The model under review builds one solid part; all positions refer to its coordinate system, in mm. Face numbers are marked on the shaded views. A direction names the side the tool comes from. Coordinates: 2 decimals unless noted, no trailing zeros. Loops run counter-clockwise (first coordinate to the right, second up) from the corner with the lowest first, then second, coordinate; pieces in that order, holes last. Notation, with made-up numbers: M 30,55.5 L 87,55.5 A23 cw 87,81.5 Z; hole C 7.5,-29.75 d9. An arc over 180 degrees is marked long. Return JSON: item names as keys, results as strings.
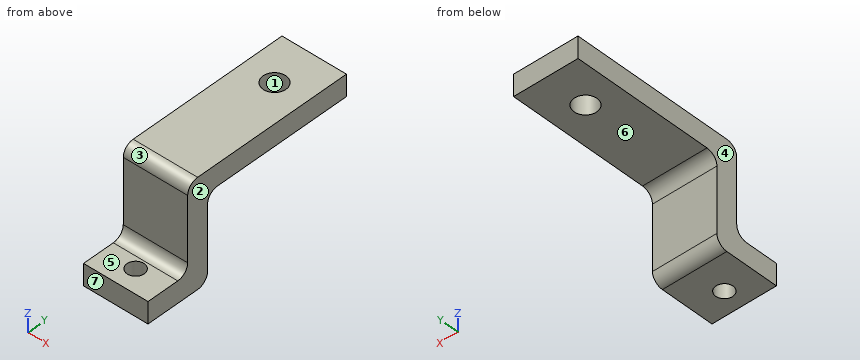
Autodesk Inventor part; units mm, degrees
ref_plane "YZ Plane" through (0, 0, 0) normal (1, 0, 0) x (0, 1, 0)
ref_plane "XZ Plane" through (0, 0, 0) normal (0, 1, 0) x (-1, 0, 0)
ref_plane "XY Plane" through (0, 0, 0) normal (0, 0, 1) x (1, 0, 0)
sketch "Sketch1" plane through (0, 0, 0) normal (1, 0, 0) x (0, 1, 0)
  line L0 (0, 0) -> (50.8, 0)
  line L1 (0, 0) -> (0, -25.4)
  line L2 (0, -25.4) -> (-12.7, -25.4)
  line L3 (50.8, -6.35) -> (6.35, -6.35)
  line L4 (6.35, -6.35) -> (6.35, -31.75)
  line L5 (6.35, -31.75) -> (-12.7, -31.75)
  line L6 (50.8, 0) -> (50.8, -6.35)
  line L7 (-12.7, -25.4) -> (-12.7, -31.75)
  dimension "d0" = 50.8
  dimension "d1" = 25.4
  dimension "d2" = 12.7
  dimension "d3" = 6.35
extrude "Extrusion1" add sketch "Sketch1" along normal blind 19.05
sketch "Sketch2" plane through (0, 0, 0) normal (0, 0, 1) x (1, 0, 0)
  line L0 (0, 50.8) -> (19.05, 50.8) construction
  line L1 (19.05, 6.35) -> (19.05, 50.8) construction
  point P0 (0, 0)
  point P1 (9.525, 38.1)
  point P2 (9.525, 50.8)
  point P3 (19.05, 28.575)
  dimension "d21" = 12.7
hole "Hole1" at (9.525, 38.1, 0) direction (0, 0, -1) diameter 6.7564 end through all
sketch "Sketch3" plane through (0, -12.7, -25.4) normal (0, 0, 1) x (1, 0, 0)
  line L0 (0, 12.7) -> (0, 0) construction
  line L1 (0, 0) -> (19.05, 0) construction
  point P0 (9.525, 6.35)
  point P1 (0, 6.35)
  point P2 (9.525, 0)
hole "Hole2" at (9.525, -6.35, -25.4) direction (0, 0, -1) diameter 5.1054 end through all
fillet "Fillet1" radius 3.175 4 edges at (9.525, 6.35, -6.35) (9.525, 0, -25.4) (9.525, 6.35, -31.75) (9.525, 0, 0)
properties part number "EL2-030" material "ABS Plastic"
1. The part is to be moulded in two halves that separate along X. For the marked faces 1, 2, 3 and 4, say which applies: released by +X, released by -X, zero draft, split by the parting line, or undercut.
Check values:
{"face 1": "undercut", "face 2": "released by +X", "face 3": "zero draft", "face 4": "released by -X"}
2. Add section B-B on x = 15.5. Give the boundary of the cut face in (y, z) (3 decimals), plus the area to 3 significant figures.
Check values:
{"outline": "M -12.7,-31.75 L 3.175,-31.75 A3.175 ccw 6.35,-28.575 L 6.35,-9.525 A3.175 cw 9.525,-6.35 L 50.8,-6.35 L 50.8,0 L 3.175,0 A3.175 ccw 0,-3.175 L 0,-22.225 A3.175 cw -3.175,-25.4 L -12.7,-25.4 Z", "area": "565 mm²"}
3. Machinability: for the marked faces 5, 6 and 7, which of the approach directions +Z, -Z, +X, -X, +Y, -Y give a long, thin tool a straight path to every point of the face, cutting with its end or side? Answer none if there is none.
Check values:
{"face 5": "+Z, +X, -X, -Y", "face 6": "-Z, +X, -X, +Y", "face 7": "+Z, -Z, +X, -X, -Y"}
4. Add section D-D on y = 46.5. Give the boundary of the cut face in (x, z).
Check values:
{"outline": "M 0,-6.35 L 19.05,-6.35 L 19.05,0 L 0,0 Z"}
5. Add section A-A on y = 38.1. Give the boundary of the cut face in (x, z).
Check values:
{"outline": "M 0,-6.35 L 6.15,-6.35 L 6.15,0 L 0,0 Z; M 12.9,-6.35 L 19.05,-6.35 L 19.05,0 L 12.9,0 Z"}
6. Insertion check: pin 1 Ø5.5 at (x, y) = (9.525, 38.1) entering from +Z; pin 2 Ø1.5 at (x, z) = (13.5, -8.5) entering from -Y; pin 3 Ø9.5 at (x, y) = (9.5, 25) entering from -Z; pin 4 Ø9.5 at (x, z) = (6.5, -18.5) entering from +Y. Each pin has a flat end and moves straight along its axis. Give the tip position at first contact, or say it passes through.
Check values:
{"pin 1": "through", "pin 2": "y = 0", "pin 3": "z = -6.35", "pin 4": "y = 6.35"}
7. To check wall thickness, follow line 1 (X direction, y = -6.35, z = -28); line 2 (Y direction, x = 3.75, z = -6); line 3 (Z direction, x = 14.5, y = 22). State the ranges of each line that lie inside material, in increasing order.
Check values:
{"line 1": "0 to 6.97, 12.08 to 19.05", "line 2": "0 to 50.8", "line 3": "-6.35 to 0"}
8. Add section C-C on y = -6.35. Give the boundary of the cut face in (x, z).
Check values:
{"outline": "M 0,-31.75 L 6.97,-31.75 L 6.97,-25.4 L 0,-25.4 Z; M 12.08,-31.75 L 19.05,-31.75 L 19.05,-25.4 L 12.08,-25.4 Z"}
